Check sheet for the modelled part. Datum: model origin and axes. Units: mm. Face numbers are marked on the shaded views. A direction names the side the tool comes from. Coordinates: 2 decimals unless noted, no trailing zeros. Write each loop counter-clockwise with the first axis right and the second up, starting at its lowest first coordinate (ties: lowest second). Pieces come first, ordered by that corner, then holes. Notation, with made-up numbers: (-6, 54.5) - (39, 54.5) arc R18 ccw to (39, 68.5) - close; hole circle Ø5 at (86, 72.5). An arc over 180 degrees is marked (long way). Write each question's results on one line, items separated by ' | '.
Autodesk Inventor part; units mm, degrees
ref_plane "YZ Plane" through (0, 0, 0) normal (1, 0, 0) x (0, 1, 0)
ref_plane "XZ Plane" through (0, 0, 0) normal (0, 1, 0) x (-1, 0, 0)
ref_plane "XY Plane" through (0, 0, 0) normal (0, 0, 1) x (1, 0, 0)
sketch "Boceto1" plane through (0, 0, 0) normal (0, 1, 0) x (-1, 0, 0)
  line L0 (0, 0) -> (-62.5, 0)
  line L1 (-62.5, 0) -> (-62.5, -75)
  line L2 (-62.5, -75) -> (0, -75)
  line L3 (0, -75) -> (0, 0)
  dimension "d0" = 62.5
  dimension "d1" = 75
extrude "Extrusión1" add sketch "Boceto1" along normal blind 3
sketch "Boceto3" plane through (0, 3, 0) normal (0, 1, 0) x (1, 0, 0)
  line L0 (0, 0) -> (62.5, 0) construction
  line L1 (31.25, 0) -> (31.25, 28) construction
  line L2 (31.25, 28) -> (0, 28)
  line L3 (0, 28) -> (0, 31)
  line L4 (0, 75) -> (0, 0)
  line L5 (0, 31) -> (62.5, 31)
  line L6 (62.5, 0) -> (62.5, 75)
  line L7 (62.5, 28) -> (31.25, 28)
  line L8 (10, 28) -> (10, 31)
  line L9 (52.5, 28) -> (52.5, 31)
  line L10 (31.25, 31) -> (31.25, 53) construction
  line L11 (31.25, 53) -> (0, 53)
  line L12 (31.25, 53) -> (62.5, 53)
  line L13 (62.5, 75) -> (0, 75) construction
  line L14 (31.25, 75) -> (31.25, 65) construction
  line L15 (62.5, 65) -> (0, 65)
  line L16 (0, 65) -> (0, 75)
  line L17 (62.5, 75) -> (62.5, 65)
  line L18 (62.5, 75) -> (0, 75)
  dimension "d4" = 28
  dimension "d5" = 3
  dimension "d9" = 22
  dimension "d10" = 10
extrude "Extrusión2" add sketch "Boceto3" along normal blind 36 contours L2 L3 L5 L8 | L9 L5 L6 L7
extrude "Extrusión3" add sketch "Boceto3" along normal blind 15 contours L2 L8 L5 L9 L7
extrude "Extrusión4" add sketch "Boceto3" along normal blind 10 contours L5 L4 L11 L12 L6
extrude "Extrusión5" add sketch "Boceto3" along normal blind 50.7 contours L4 L18 L6 L15
sketch "Boceto4" plane through (0, 3, -28) normal (0, 0, 1) x (1, 0, 0)
  line L0 (62.5, 0) -> (0, 0) construction
  line L1 (62.5, 0) -> (62.5, 36) construction
  line L2 (52.5, 36) -> (62.5, 36) construction
  line L3 (52.5, 15) -> (52.5, 36) construction
  line L4 (10, 15) -> (52.5, 15) construction
  line L5 (10, 15) -> (10, 36) construction
  line L6 (0, 36) -> (10, 36) construction
  line L7 (0, 0) -> (0, 36) construction
  line L8 (0, 0) -> (0, 22) construction
  line L9 (0, 0) -> (0, 32) construction
  line L10 (0, -3) -> (0, 19) construction
  line L11 (0, 19) -> (62.5, 19) construction
  line L12 (0, -3) -> (0, 29) construction
  line L13 (0, 29) -> (62.5, 29) construction
  line L14 (0, 29) -> (6.25, 29) construction
  line L15 (0, 19) -> (6.25, 19) construction
  line L16 (62.5, 29) -> (56.25, 29) construction
  line L17 (62.5, 19) -> (56.25, 19) construction
  circle A0 centre (6.25, 29) radius 2
  circle A1 centre (6.25, 19) radius 2
  line L18 (62.5, -3) -> (0, -3) construction
  line L19 (31.25, -3) -> (31.25, 50.7118) construction
  circle A2 centre (56.25, 29) radius 2
  circle A3 centre (56.25, 19) radius 2
  dimension "d21" = 22
  dimension "d22" = 32
  dimension "d23" = 6.25
  dimension "d24" = 6.25
  dimension "d25" = 6.25
  dimension "d26" = 4
  dimension "d27" = 4
extrude "Extrusión6" cut sketch "Boceto4" against normal blind 20
sketch "Boceto5" plane through (0, 3, -65) normal (0, 0, 1) x (1, 0, 0)
  line L0 (62.5, -3) -> (0, -3) construction
  line L1 (0, -3) -> (0, 25) construction
  line L2 (0, 10) -> (0, 36) construction
  line L3 (0, -3) -> (40.5, -3) construction
  line L4 (40.5, -3) -> (40.5, 25) construction
  circle A0 centre (40.5, 25) radius 2.5
  dimension "d30" = 28
  dimension "d31" = 40.5
  dimension "d32" = 5
extrude "Extrusión7" cut sketch "Boceto5" against normal blind 20
properties part number "Mounting2"
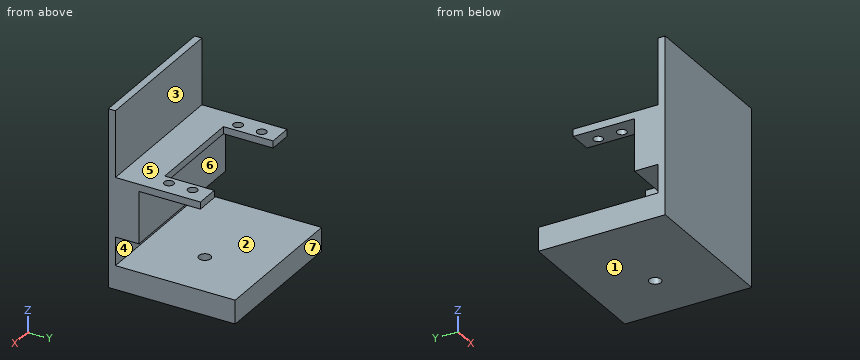
1. Access from +Z, -Z, +X, -X, +Y, -Y to the whole of each face (thin tool, end or side, straight path). Record for the marked faces 1, 2 and 3.
Values follow:
face 1: -Z, +X, -X, +Y, -Y | face 2: +X, -X, +Y | face 3: +Z, +X, -X, +Y
2. Sectioned sample at C-C (x = 56.25). Record the cut outline in (y, z), then the cut area to 3 significant figures.
Values follow:
outline: (0, -75) - (53.7, -75) - (53.7, -65) - (3, -65) - (3, -53) - (13, -53) - (13, -31) - (20, -31) - (20, -28) - (3, -28) - (3, 0) - (0, 0) - close; (24, -31) - (30, -31) - (30, -28) - (24, -28) - close; (34, -31) - (39, -31) - (39, -28) - (34, -28) - close | area: 1,040 mm^2
3. Material ranges on L1, parallel to Y at x = 6.25, z = -29.75; L2, parallel to Z at x = 5.5, y = 35; L3, parallel to Z at x = 18, y = 44, recorded low to high. Write a range as [from, to].
Values follow:
L1: y = [0, 20], [24, 30], [34, 39] | L2: z = [-75, -65], [-31, -28] | L3: z = [-75, -65]
4. Sectioned sample at A-A (x = 40.5). Record the cut outline in (y, z), then the cut area to 3 significant figures.
Values follow:
outline: (0, -75) - (25.5, -75) - (25.5, -65) - (3, -65) - (3, -53) - (13, -53) - (13, -31) - (18, -31) - (18, -28) - (3, -28) - (3, 0) - (0, 0) - close; (30.5, -75) - (53.7, -75) - (53.7, -65) - (30.5, -65) - close | area: 947 mm^2
5. Draft check along Z on the marked faces 4, 5, 6 and 7. Enter one of: pulls with the +Z half, pulls with the -Z half, needs draft (parallel to the pull), parting line crosses it, or undercut.
Values follow:
face 4: undercut | face 5: pulls with the +Z half | face 6: undercut | face 7: needs draft
6. Sectioned sample at B-B (y = 28). Record the cut outline in (x, z), then the cut area to 3 significant figures.
Values follow:
outline: (0, -75) - (38, -75) - (38, -65) - (0, -65) - close; (0, -31) - (10, -31) - (10, -28) - (0, -28) - close; (43, -75) - (62.5, -75) - (62.5, -65) - (43, -65) - close; (52.5, -31) - (62.5, -31) - (62.5, -28) - (52.5, -28) - close | area: 635 mm^2
7. Sectioned sample at D-D (x = 13). Record the cut outline in (y, z), then the cut area to 3 significant figures.
Values follow:
outline: (0, -75) - (53.7, -75) - (53.7, -65) - (3, -65) - (3, -53) - (13, -53) - (13, -31) - (18, -31) - (18, -28) - (3, -28) - (3, 0) - (0, 0) - close | area: 997 mm^2
8. Go/stop test with flat-tipped pins: pin 1 (2.5 mm diameter, centred on x = 56.25, y = 32, fed in from +Z); pin 2 (2.5 mm diameter, centred on x = 58.5, z = -30, fed in from +Y); pin 3 (3 mm diameter, centred on x = 52, z = -62.5, fed in from +Y). Record where each tip stops, or that it passes through.
Values follow:
pin 1: stops at z = -65 | pin 2: stops at y = 39 | pin 3: stops at y = 3
